The model under review builds one solid part; all positions refer to its coordinate system, in mm. A direction names the side the tool comes from. Give positions to 0.01 mm unless a question says otherwise; leave off trailing zeros. Loops run counter-clockwise (first coordinate to the right, second up) from the corner with the lowest first, then second, coordinate; pieces in that order, holes last. Notation, with made-up numbers: M 22.25,72 L 41.25,72 A36 ccw 41.25,110 Z; hole C 76,41.5 d10. An arc over 180 degrees is marked long. Return JSON: item names as keys, results as strings. Group by question number.
```python
from build123d import *

# Parameters (mm, degrees)
CUT_EXTRUDE_1_DEPTH = 2.5
FILLET_1_R          = 0.3
CHAMFER_1_SIZE      = 1.6


with BuildPart() as part:
    # Эскиз1 → Повернуть1 (revolve)
    with BuildSketch(Plane.XY):
        Polygon((0, 0), (0, 6.5), (8, 6.5), (8, 4), (33, 4), (33, 0), align=None)
    revolve(axis=Axis((33, 0, 0), (-1, 0, 0)))

    # Эскиз2 → Вырез-Вытянуть1 (cut)
    with BuildSketch(Plane.ZY):
        Polygon((-1.732050808, 3), (-3.464101615, 0), (-1.732050808, -3), (1.732050808, -3), (3.464101615, 0), (1.732050808, 3), align=None)
    extrude(amount=-CUT_EXTRUDE_1_DEPTH, mode=Mode.SUBTRACT)

    # Скругление1
    fillet_1_edges = [part.edges().sort_by_distance(p)[0] for p in [
        (8, -4, 0),
        (0, -6.5, 0),
    ]]
    fillet(fillet_1_edges, radius=FILLET_1_R)

    # Фаска1
    chamfer_1_edges = [part.edges().sort_by_distance(p)[0] for p in [
        (33, -4, 0),
    ]]
    chamfer(chamfer_1_edges, length=CHAMFER_1_SIZE)


solid = part.part
```
(1) Add section A-A (z = 0). Write out the cut boundary in (x, y).
(2) Mouldability with a two-part tool opening along Z and no side actions: class faces 4 (the flat face through (0, 1.5, -2.8)), 5 (the flat face through (1.2, 1.5, 2.6)), 6 (the cylindrical face through (20.012, -0.867, 3.905)) as released by +Z, released by -Z, zero draft, split by the parting line, or undercut.
(3) For probe 1 along X at (y, z) = (3.5, 2.5); probe 2 along X at (y, z) = (0, -0.75); probe 3 along Y at (x, z) = (8.5, 0), list the stretches that pass through material, from the lowest coordinate up.
(4) For faces 1 (the cylindrical face through (4.204, -5.158, 3.955)), 2 (the flat face through (8, 1.353, 4.242)), 3 (the flat face through (1, -3, 0)), list the 3-axis set-ups (+Z, -Z, +X, -X, +Y, -Y) from which the entire face can be reached by the end or side of a thin tool; tool diameter is ignored.
(5) For pin 1 (1 mm diameter, centred on x = 6, y = -1, fed in from +Z); pin 2 (6.5 mm diameter, centred on y = 0, z = -1.5, fed in from -X); pin 3 (2 mm diameter, centred on x = 24, z = -3, fed in from -Y); pin 4 (2 mm diameter, centred on x = 23.5, y = 0, fed in from -Z), all flat-tipped, find the tip position at first contact; note any pin that passes through.
(6) Add section B-B (x = 9). Write out the cut boundary in (y, z).
Verdict:
{
 "1": {"outline": "M 0,-6.2 A0.3 ccw 0.3,-6.5 L 8,-6.5 L 8,-4.3 A0.3 cw 8.3,-4 L 31.4,-4 L 33,-2.4 L 33,2.4 L 31.4,4 L 8.3,4 A0.3 cw 8,4.3 L 8,6.5 L 0.3,6.5 A0.3 ccw 0,6.2 L 0,3 L 2.5,3 L 2.5,-3 L 0,-3 Z"},
 "2": {"face 4": "zero draft", "face 5": "undercut", "face 6": "split by the parting line"},
 "3": {"probe 1": "x = 0 to 8", "probe 2": "x = 2.5 to 33", "probe 3": "y = -4 to 4"},
 "4": {"face 1": "+X, -X", "face 2": "+X", "face 3": "-X"},
 "5": {"pin 1": "stops at z = 6.48", "pin 2": "stops at x = 0", "pin 3": "stops at y = -3.46", "pin 4": "stops at z = -4"},
 "6": {"outline": "C 0,0 d8"}
}
